Design review of the part shown in the three views and the two pictorial views. Dimensions are in mm from the part's minimum x, y and z. A direction names the side the tool comes from. Coordinates: 2 decimals unless noted, no trailing zeros. Write each loop counter-clockwise with the first axis right and the second up, starting at its lowest first coordinate (ties: lowest second). Pieces come first, ordered by that corner, then holes. Notation, with made-up numbers: (63.5, -11.75) -> (122.5, -11.75) arc R13 ccw to (122.5, 13.25) -> close; hole circle Ø8 at (-21.5, 84.25). An arc over 180 degrees is marked (long way). Write each question's results on one line, items separated by ' | '.
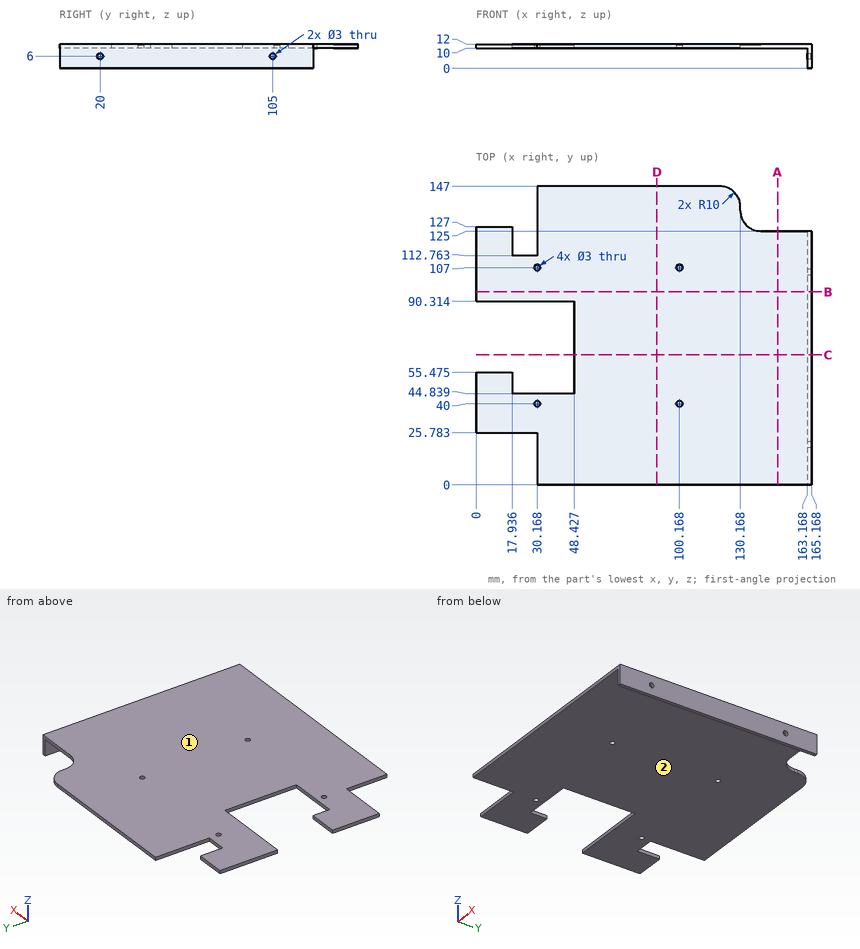
Q1. Add section A-A (x = 148.5). Write out the cut boundary in (y, z), plus the area to 3 significant figures.
Solution:
outline: (0, 10) -> (125, 10) -> (125, 12) -> (0, 12) -> close | area: 250 mm²
Q2. Add section C-C (y = 64). Write out the cut boundary in (x, z).
Solution:
outline: (48.43, 10) -> (163.17, 10) -> (163.17, 0) -> (165.17, 0) -> (165.17, 12) -> (48.43, 12) -> close
Q3. For line 1 (X direction, y = 40, z = 10.7); line 2 (Y direction, x = 164.6, z = 6); line 3 (Z direction, x = 163.9, y = 105), list the stretches that pass through material, from the lowest coordinate up. Write a range as from..to.
Solution:
line 1: 0..28.67, 31.67..98.67, 101.67..165.17 | line 2: 0..18.5, 21.5..103.5, 106.5..125 | line 3: 0..4.5, 7.5..12
Q4. Clearance check with flat-ended pins moving along their axes: P1, Ø1, axis at x = 12, z = 11, coming from the +Y side; P2, Ø2, axis at y = 28, z = 5, coming from the -X side; P3, Ø2, axis at x = 22, z = 10.5, coming from the -Y side. State where each tip first meets the part, or that it passes through.
Solution:
P1: y = 127 | P2: x = 163.17 | P3: y = 25.78
Q5. Add section B-B (y = 95). Write out the cut boundary in (x, z).
Solution:
outline: (0, 10) -> (163.17, 10) -> (163.17, 0) -> (165.17, 0) -> (165.17, 12) -> (0, 12) -> close
Q6. Add section D-D (x = 89). Write out the cut boundary in (y, z), plus the area to 3 significant figures.
Solution:
outline: (0, 10) -> (147, 10) -> (147, 12) -> (0, 12) -> close | area: 294 mm²
Q7. Machinability: for the marked faces 1 and 2, which of the approach directions +Z, -Z, +X, -X, +Y, -Y give a long, thin tool a straight path to every point of the face, cutting with its end or side? Answer none if there is none.
Solution:
face 1: +Z, +X, -X, +Y, -Y | face 2: -Z, -X, +Y, -Y
